For this review, take the finished solid that the model builds, in its own axes (mm). Face numbers are marked on the shaded views. Give positions to 0.01 mm unless a question says otherwise; leave off trailing zeros. Loops run counter-clockwise (first coordinate to the right, second up) from the corner with the lowest first, then second, coordinate; pieces in that order, holes last.
```python
from build123d import *

# Parameters (mm, degrees)
F1_DEPTH = 3.5
F2_R     = 11
F3_DEPTH = 63.5
F5_DEPTH = 6.35


with BuildPart() as f1:
    # F0 (on Top) → F1 (new body, symmetric)
    with BuildSketch(Plane.XY):
        with BuildLine():
            Line((20.552645, -35.598226), (41.713538, -35.598226))
            Line((41.713538, -35.598226), (51.685737, -18.325871))
            Line((51.685737, -18.325871), (41.105291, 0))
            ThreePointArc((41.105291, 0), (19.628403, 11.332464), (20.552645, 35.598226))
            Line((20.552645, 35.598226), (9.972199, 53.924097))
            Line((9.972199, 53.924097), (-9.972199, 53.924097))
            Line((-9.972199, 53.924097), (-20.552645, 35.598226))
            ThreePointArc((-20.552645, 35.598226), (-19.628403, 11.332464), (-41.105291, 0))
            Line((-41.105291, 0), (-51.685737, -18.325871))
            Line((-51.685737, -18.325871), (-41.713538, -35.598226))
            Line((-41.713538, -35.598226), (-20.552645, -35.598226))
            ThreePointArc((-20.552645, -35.598226), (0, -22.664928), (20.552645, -35.598226))
        make_face()
    extrude(amount=F1_DEPTH, both=True)

    # F2 (on face) → F3 (cut)
    with BuildSketch(Plane.XY.offset(3.5)):
        Circle(F2_R)
    extrude(amount=-F3_DEPTH, mode=Mode.SUBTRACT)

    # F4 (on Top) → F5 (join, symmetric)
    with BuildSketch(Plane.XY):
        Polygon((8.473816, 51.294833), (-8.925753, 51.294833), (-13.671091, 21.692971), (13.671093, 21.692971), align=None)
        Polygon((-11.951118, -22.685997), (-25.62221, 0.993028), (-48.659537, -18.308877), (-39.959752, -33.377345), align=None)
        Polygon((25.622209, 0.993027), (11.951117, -22.685999), (40.185721, -32.985957), (48.885505, -17.917488), align=None)
    extrude(amount=F5_DEPTH, both=True)


solid = f1.part
```
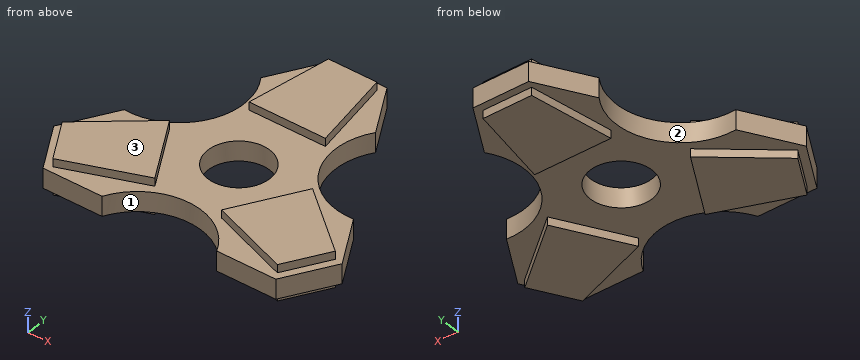
Q1. Consider section D-D on x = 32. Give the boundary of the cut face in (y, z).
Answers:
outline: (-35.6, -3.5) - (-30, -3.5) - (-30, -6.35) - (-4.19, -6.35) - (-4.19, -3.5) - (1.16, -3.5) - (1.16, 3.5) - (-4.19, 3.5) - (-4.19, 6.35) - (-30, 6.35) - (-30, 3.5) - (-35.6, 3.5) - close
Q2. Mouldability with a two-part tool opening along Y and no side actions: class the marked faces 1, 2 and 3 as +Y half, -Y half, draft (parallel to the pull), parting line (faces both ways), or undercut.
Answers:
face 1: -Y half
face 2: undercut
face 3: draft
Q3. For pin 1 Ø3 at (x, z) = (-1, 5.5) entering from +Y; pin 2 Ø0.9 at (x, z) = (-7, 4) entering from -Y; pin 3 Ø1.5 at (y, z) = (-3, -1.5) entering from -X, all flat-tipped, find the tip position at first contact; note any pin that passes through.
Answers:
pin 1: stops at y = 51.29
pin 2: stops at y = 21.69
pin 3: stops at x = -43.27
Q4. For probe 1 along Y at (x, z) = (0, 1.5); probe 2 along Z at (x, y) = (4, 13.5); probe 3 along X at (y, z) = (-8, 5.75), list the stretches that pass through material, from the lowest coordinate up.
Answers:
probe 1: y = -22.66 to -11, 11 to 53.92
probe 2: z = -3.5 to 3.5
probe 3: x = -36.36 to -20.43, 20.43 to 36.69
Q5. Consider section A-A on x = 0. Give the boundary of the cut face in (y, z), plus the area to 3 significant figures.
Answers:
outline: (-22.66, -3.5) - (-11, -3.5) - (-11, 3.5) - (-22.66, 3.5) - close; (11, -3.5) - (21.69, -3.5) - (21.69, -6.35) - (51.29, -6.35) - (51.29, -3.5) - (53.92, -3.5) - (53.92, 3.5) - (51.29, 3.5) - (51.29, 6.35) - (21.69, 6.35) - (21.69, 3.5) - (11, 3.5) - close
area: 551 mm2
Q6. Consider section B-B on y = 5. Give the boundary of the cut face in (x, z).
Answers:
outline: (-25.04, -3.5) - (-9.8, -3.5) - (-9.8, 3.5) - (-25.04, 3.5) - close; (9.8, -3.5) - (25.04, -3.5) - (25.04, 3.5) - (9.8, 3.5) - close
Q7. Consider section C-C on z = 0. Give the boundary of the cut face in (x, y), plus the area to 3 significant figures.
Answers:
outline: (-51.69, -18.33) - (-41.71, -35.6) - (-20.55, -35.6) arc R22.8 cw to (20.55, -35.6) - (41.71, -35.6) - (51.69, -18.33) - (41.11, 0) arc R22.8 cw to (20.55, 35.6) - (9.97, 53.92) - (-9.97, 53.92) - (-20.55, 35.6) arc R22.8 cw to (-41.11, 0) - close; hole circle Ø22 at (0, 0)
area: 4,540 mm2
